Design review of the part shown in the three views and the two pictorial views. Dimensions are in mm from the part's minimum x, y and z. Give positions to 0.01 mm unless a question says otherwise; leave off trailing zeros. Write each loop counter-clockwise with the first axis right and the second up, starting at its lowest first coordinate (ties: lowest second). Pieces come first, ordered by that corner, then holes. Notation, with made-up numbers: M -38.5,-19 L -21.5,-19 A20 ccw -21.5,16 Z; hole C 17,28 d6. An arc over 180 degrees is marked long. Use one line per item in the form item = value. Start each with the question number.
Q1. Consider section C-C on x = 9. Write out the cut boundary in (y, z), and give its area (3 significant figures).
Q2. Consider section A-A on z = 13.25. Write out the cut boundary in (x, y) (1 decimal).
Q3. Clearance check with flat-ended pins moving along their axes: pin 1 Ø8 at (y, z) = (15, 5) entering from +X (1 decimal); pin 2 Ø3 at (x, z) = (18.5, 11) entering from +Y (1 decimal); pin 3 Ø4 at (x, z) = (12.5, 18.5) entering from +Y (1 decimal). State where each tip first meets the part, or that it passes through.
Q4. Mouldability with a two-part tool opening along Y and no side actions: class the marked faces 1, 2, 3 and 4 as released by +Y, released by -Y, zero draft, split by the parting line, or undercut.
Q5. For probe 1 along X at (y, z) = (6.5, 9) (1 decimal); probe 2 along Y at (x, z) = (7, 12.5) (1 decimal); probe 3 along Y at (x, z) = (9, 12.25) (1 decimal), list the stretches that pass through material, from the lowest coordinate up. Write a range as [from, to].
Q6. Consider section D-D on x = 16.5. Write out the cut boundary in (y, z).
Q7. Consider section B-B on y = 8. Write out the cut boundary in (x, z), and give its area (3 significant figures).
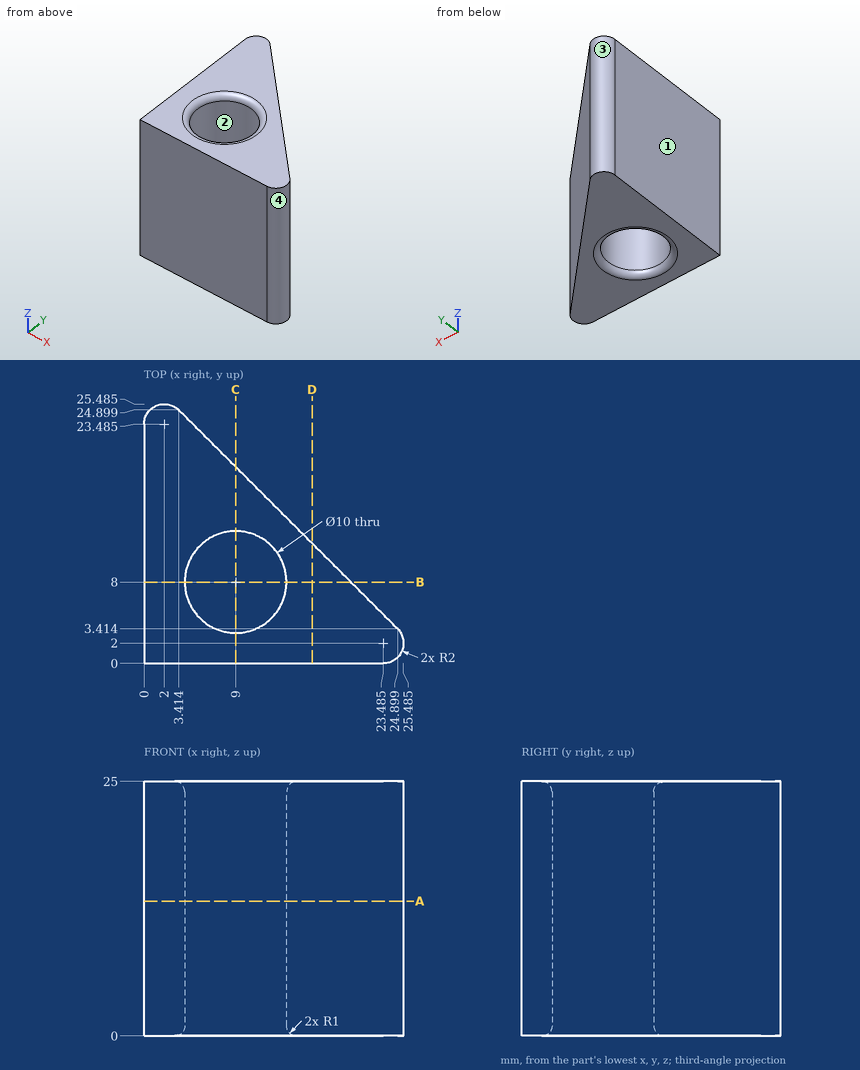
Working result:
q1.outline = M 0,0 L 2,0 A1 ccw 3,1 L 3,24 A1 ccw 2,25 L 0,25 Z; M 13,1 A1 ccw 14,0 L 19.31,0 L 19.31,25 L 14,25 A1 ccw 13,24 Z
q1.area = 232 mm²
q2.outline = M 0,0 L 23.5,0 A2 ccw 24.9,3.4 L 3.4,24.9 A2 ccw 0,23.5 Z; hole C 9,8 d10
q3.pin_1 = 17.3
q3.pin_2 = 11.3
q3.pin_3 = 17.8
q4.face_1 = zero draft
q4.face_2 = undercut
q4.face_3 = released by +Y
q4.face_4 = split by the parting line
q5.probe_1 = [0, 4.2], [13.8, 21.8]
q5.probe_2 = [0, 3.4], [12.6, 21.3]
q5.probe_3 = [0, 3], [13, 19.3]
q6.outline = M 0,0 L 11.81,0 L 11.81,25 L 0,25 Z
q7.outline = M 0,0 L 3,0 A1 ccw 4,1 L 4,24 A1 ccw 3,25 L 0,25 Z; M 14,1 A1 ccw 15,0 L 20.31,0 L 20.31,25 L 15,25 A1 ccw 14,24 Z
q7.area = 257 mm²
